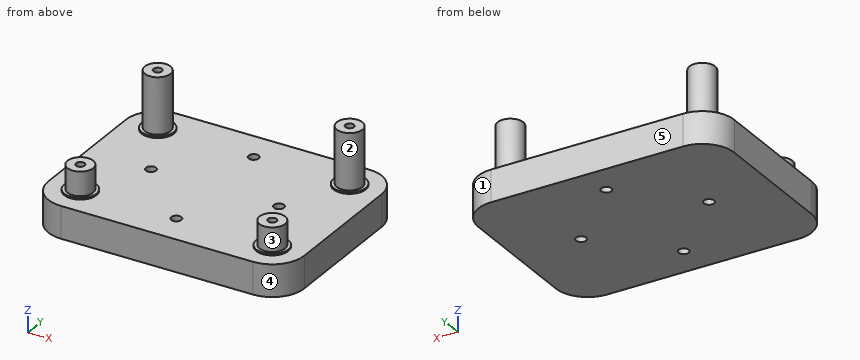
```python
from build123d import *

# Parameters (mm, degrees)
SKETCH1_W               = 80
SKETCH1_H               = 60
BOSS_EXTRUDE1_DEPTH     = 10
SKETCH1_3_R             = 4.025
SKETCH1_3_R_2           = 1.35
BOSS_EXTRUDE2_DEPTH     = 8
SKETCH1_5_R             = 4.025
SKETCH1_5_R_2           = 1.35
BOSS_EXTRUDE4_DEPTH     = 18
SKETCH1_4_R             = 5.025
SKETCH1_4_R_2           = 4.025
BOSS_EXTRUDE3_DEPTH     = 0.5
SKETCH1_6_R             = 1.6
CUT_EXTRUDE1_DEPTH      = 19
CUT_EXTRUDE1_DEPTH_BACK = 11
FILLET1_R               = 10


with BuildPart() as part:
    # Sketch1 → Boss-Extrude1 (new body)
    with BuildSketch(Plane.XY):
        Rectangle(SKETCH1_W, SKETCH1_H)
    extrude(amount=-BOSS_EXTRUDE1_DEPTH)

    # Sketch1<3> → Boss-Extrude2 (add)
    with BuildSketch(Plane.XY):
        with Locations((-30, -20)):
            Circle(SKETCH1_3_R)
        with Locations((-30, -20)):
            Circle(SKETCH1_3_R_2, mode=Mode.SUBTRACT)
        with Locations((30, -20)):
            Circle(SKETCH1_3_R)
        with Locations((30, -20)):
            Circle(SKETCH1_3_R_2, mode=Mode.SUBTRACT)
    extrude(amount=BOSS_EXTRUDE2_DEPTH)

    # Sketch1<5> → Boss-Extrude4 (add)
    with BuildSketch(Plane.XY):
        with Locations((-30, 20)):
            Circle(SKETCH1_5_R)
        with Locations((-30, 20)):
            Circle(SKETCH1_5_R_2, mode=Mode.SUBTRACT)
        with Locations((30, 20)):
            Circle(SKETCH1_5_R)
        with Locations((30, 20)):
            Circle(SKETCH1_5_R_2, mode=Mode.SUBTRACT)
    extrude(amount=BOSS_EXTRUDE4_DEPTH)

    # Sketch1<4> → Boss-Extrude3 (add)
    with BuildSketch(Plane.XY):
        with Locations((-30, 20)):
            Circle(SKETCH1_4_R)
        with Locations((-30, 20)):
            Circle(SKETCH1_4_R_2, mode=Mode.SUBTRACT)
        with Locations((30, 20)):
            Circle(SKETCH1_4_R)
        with Locations((30, 20)):
            Circle(SKETCH1_4_R_2, mode=Mode.SUBTRACT)
        with Locations((30, -20)):
            Circle(SKETCH1_4_R)
        with Locations((30, -20)):
            Circle(SKETCH1_4_R_2, mode=Mode.SUBTRACT)
        with Locations((-30, -20)):
            Circle(SKETCH1_4_R)
        with Locations((-30, -20)):
            Circle(SKETCH1_4_R_2, mode=Mode.SUBTRACT)
    extrude(amount=BOSS_EXTRUDE3_DEPTH)

    # Sketch1<6> → Cut-Extrude1 (cut, two sides)
    with BuildSketch(Plane.XY) as cut_extrude1_sk:
        with Locations((0, 20)):
            Circle(SKETCH1_6_R)
        with Locations((-20, 0)):
            Circle(SKETCH1_6_R)
        with Locations((0, -20)):
            Circle(SKETCH1_6_R)
        with Locations((20, 0)):
            Circle(SKETCH1_6_R)
    extrude(amount=CUT_EXTRUDE1_DEPTH, mode=Mode.SUBTRACT)
    extrude(cut_extrude1_sk.sketch, amount=-CUT_EXTRUDE1_DEPTH_BACK, mode=Mode.SUBTRACT)

    # Fillet1
    fillet1_edges = [part.edges().sort_by_distance(p)[0] for p in [
        (-40, 30, -5),
        (-40, -30, -5),
        (40, -30, -5),
        (40, 30, -5),
    ]]
    fillet(fillet1_edges, radius=FILLET1_R)


solid = part.part
```
Design review of the part built by this model. Coordinates are the model's own, in mm. Face numbers are marked on the shaded views. A direction names the side the tool comes from. Give positions to 0.01 mm unless a question says otherwise; leave off trailing zeros. Order: outer loops, then holes, each group sorted by start corner. A loop starts at its lowest first (then second) coordinate and runs counter-clockwise, first axis right, second up. Notation, with made-up numbers: (33.5, 60.5) - (48.5, 60.5) arc R23 cw to (48.5, 95.5) - close; hole circle Ø3 at (-30.5, 10.25). An arc over 180 degrees is marked (long way). Use a Markdown table: item, result. Add a question column.
(1) Add section D-D on y = 17. Give the boundary of the cut face in (x, z).
(2) Add section B-B on y = 0. Give the boundary of the cut face in (x, z), then the cut area to 3 significant figures.
(3) Add section C-C on z = -4.25. Give the boundary of the cut face in (x, y).
(4) Machinability: for the marked faces 1 and 2, which of the approach directions +Z, -Z, +X, -X, +Y, -Y give a long, thin tool a straight path to every point of the face, cutting with its end or side? Answer none if there is none.
(5) Mouldability with a two-part tool opening along Y and no side actions: class the marked faces 3, 4 and 5 as +Y half, -Y half, draft (parallel to the pull), parting line (faces both ways), or undercut.
(6) Add section A-A on x = -20. Give the boundary of the cut face in (y, z), then the cut area to 3 significant figures.
(7) Wall thickness on probe 1 along Y at (x, z) = (0, -3.25); probe 2 along Y at (x, z) = (-30, 4.75) (3 decimals); probe 3 along Y at (x, z) = (-30, 14) (3 decimals): over which ranges is each line inside the solid? List them lowest first. Write a range as [from, to].
(8) Clearance check with flat-ended pins moving along their axes: P1, Ø0.8, axis at x = -29.5, y = 20, coming from the +Z side; P2, Ø1.4, axis at x = -30.5, y = -20.5, coming from the +Z side; P3, Ø12, axis at y = 5, z = 14.5, coming from the -X side; P4, Ø8, axis at x = 22.5, z = 14.5, coming from the +Y side. State where each tip first meets the part, or that it passes through.
Report:
| question | item | result |
|---|---|---|
| 1 | outline | (-40, -10) - (40, -10) - (40, 0) - (34.03, 0) - (34.03, 0.5) - (32.68, 0.5) - (32.68, 18) - (27.32, 18) - (27.32, 0.5) - (25.97, 0.5) - (25.97, 0) - (-25.97, 0) - (-25.97, 0.5) - (-27.32, 0.5) - (-27.32, 18) - (-32.68, 18) - (-32.68, 0.5) - (-34.03, 0.5) - (-34.03, 0) - (-40, 0) - close |
| 2 | outline | (-40, -10) - (-21.6, -10) - (-21.6, 0) - (-40, 0) - close; (-18.4, -10) - (18.4, -10) - (18.4, 0) - (-18.4, 0) - close; (21.6, -10) - (40, -10) - (40, 0) - (21.6, 0) - close |
| 2 | area | 736 mm² |
| 3 | outline | (-40, -20) arc R10 ccw to (-30, -30) - (30, -30) arc R10 ccw to (40, -20) - (40, 20) arc R10 ccw to (30, 30) - (-30, 30) arc R10 ccw to (-40, 20) - close; hole circle Ø3.2 at (-20, 0); hole circle Ø3.2 at (0, -20); hole circle Ø3.2 at (0, 20); hole circle Ø3.2 at (20, 0) |
| 4 | face 1 | +Z, -Z, +X, +Y |
| 4 | face 2 | +Z |
| 5 | face 3 | undercut |
| 5 | face 4 | -Y half |
| 5 | face 5 | +Y half |
| 6 | outline | (-30, -10) - (-1.6, -10) - (-1.6, 0) - (-30, 0) - close; (1.6, -10) - (30, -10) - (30, 0) - (1.6, 0) - close |
| 6 | area | 568 mm² |
| 7 | probe 1 | y = [-30, -21.6], [-18.4, 18.4], [21.6, 30] |
| 7 | probe 2 | y = [-24.025, -21.35], [-18.65, -15.975], [15.975, 18.65], [21.35, 24.025] |
| 7 | probe 3 | y = [15.975, 18.65], [21.35, 24.025] |
| 8 | P1 | stops at z = 0 |
| 8 | P2 | stops at z = 8 |
| 8 | P3 | passes through |
| 8 | P4 | stops at y = 21.99 |
